Verification items for the finished model (mm, model axes). A direction names the side the tool comes from. Coordinates: 2 decimals unless noted, no trailing zeros. Write each loop counter-clockwise with the first axis right and the second up, starting at its lowest first coordinate (ties: lowest second). Pieces come first, ordered by that corner, then holes. Notation, with made-up numbers: M 46,42 L 95,42 A18 ccw 95,63 Z; hole C -29.5,73 d2. An arc over 180 degrees is marked long. Answer in a Markdown table with one row per item.
from build123d import *

# Parameters (mm, degrees)
PAD_DEPTH    = 11
SKETCH001_R  = 1
PAD001_DEPTH = 9.5
POCKET_DEPTH = 2.5


with BuildPart() as part:
    # Sketch → Pad (new body)
    with BuildSketch(Plane.XY):
        with BuildLine():
            Line((-1.5, 1.486438), (-1.5, -1.486438))
            Line((-1.5, -1.486438), (-0.5, -1.486438))
            Line((-0.5, -1.486438), (-0.5, -1.836438))
            Line((-0.5, -1.836438), (0.5, -1.836438))
            Line((0.5, -1.836438), (0.5, -1.486438))
            Line((0.5, -1.486438), (1.5, -1.486438))
            Line((1.5, -1.486438), (1.5, 1.486438))
            ThreePointArc((1.5, 1.486438), (0, 2.163562), (-1.5, 1.486438))
        make_face()
    extrude(amount=PAD_DEPTH)

    # Sketch001 → Pad001 (join, symmetric)
    with BuildSketch(Plane.YZ):
        with Locations((0.338562, 0)):
            Circle(SKETCH001_R)
    extrude(amount=PAD001_DEPTH, both=True)

    # Sketch002 → Pocket (cut, symmetric)
    with BuildSketch(Plane.YZ):
        with BuildLine():
            ThreePointArc((-1.836438, 2), (-1.397096, 0.912957), (-0.661438, 0))
            Line((-3.011438, 0), (-0.661438, 0))
            Line((-3.011438, 2), (-3.011438, 0))
            Line((-1.836438, 2), (-3.011438, 2))
        make_face()
        with BuildLine():
            ThreePointArc((1.338562, 0), (1.888846, 0.943164), (2.163562, 2))
            Line((2.163562, 2), (3.338562, 2))
            Line((3.338562, 2), (3.338562, 0))
            Line((3.338562, 0), (1.338562, 0))
        make_face()
    extrude(amount=POCKET_DEPTH, both=True, mode=Mode.SUBTRACT)


solid = part.part
1) Depth check by flat-ended pin: pin 1 (6 mm diameter, centred on x = 6.5, z = 6.5, fed in from -Y); pin 2 (0.5 mm diameter, centred on x = 1, z = 7.5, fed in from -Y); pin 3 (2 mm diameter, centred on x = 6, y = -1, fed in from +Z); pin 4 (0.9 mm diameter, centred on y = 0.5, z = 5, fed in from -X). Enter the tip coordinate at first touch or a pass-through.
Response values:
| item | result |
|---|---|
| pin 1 | passes through |
| pin 2 | stops at y = -1.49 |
| pin 3 | stops at z = 0.94 |
| pin 4 | stops at x = -1.5 |
2) Thickness scan on L1, parallel to X at y = 1.3, z = 3; L2, parallel to X at y = -1.6, z = 5.5; L3, parallel to Y at x = 7.5, z = 0. Record the ranges inside material, lowest first. Write a range as [from, to].
Response values:
| item | result |
|---|---|
| L1 | x = [-1.5, 1.5] |
| L2 | x = [-0.5, 0.5] |
| L3 | y = [-0.66, 1.34] |
3) Sectioned sample at B-B (y = 1.1). Record the cut outline in (x, z), then the cut area to 3 significant figures.
Response values:
| item | result |
|---|---|
| outline | M -9.5,-0.65 L 9.5,-0.65 L 9.5,0.65 L 1.5,0.65 L 1.5,11 L -1.5,11 L -1.5,0.65 L -9.5,0.65 Z |
| area | 55.7 mm² |
4) Sectioned sample at A-A (z = 8.5). Record the cut outline in (x, y).
Response values:
| item | result |
|---|---|
| outline | M -1.5,-1.49 L -0.5,-1.49 L -0.5,-1.84 L 0.5,-1.84 L 0.5,-1.49 L 1.5,-1.49 L 1.5,1.49 A2 ccw -1.5,1.49 Z |
5) Tool access check on faces 1 (the face through (0.021, 1.783, 0.708)), 2 (the face through (-1, -1.486, 6)), 3 (the face through (1, -1.486, 6)), 4 (the face through (0.133, 0.122, -0.976)). Record the directions out of +Z, -Z, +X, -X, +Y, -Y that give a thin tool (end or side, any length) a straight path to the whole face; none if there is none.
Response values:
| item | result |
|---|---|
| face 1 | -Z, +X, -X, +Y |
| face 2 | +Z, -Z, -X, -Y |
| face 3 | +Z, -Z, +X, -Y |
| face 4 | none |
6) Sectioned sample at C-C (x = -4.25). Record the cut outline in (y, z), then the cut area to 3 significant figures.
Response values:
| item | result |
|---|---|
| outline | C 0.34,0 d2 |
| area | 3.14 mm² |
